Could you check a few things on this drawing? It's one solid part, dimensions in mm from its lowest x, y, z. Coordinates: 2 decimals unless noted, no trailing zeros. Write each loop counter-clockwise with the first axis right and the second up, starting at its lowest first coordinate (ties: lowest second). Pieces come first, ordered by that corner, then holes.
Item 1: I want a section at C-C (z = 1.65). Please give me the cut outline in (x, y), and give its area (3 significant figures).
Item 2: I'm going to push flat-ended pins straight in: P1, Ø1.5, axis at y = 20, z = 0.5, coming from the -X side; P2, Ø2.5, axis at x = 21.4, y = 21.4, coming from the +Z side; P3, Ø6, axis at x = 13, y = 15, coming from the -Z side; P4, Ø1, axis at y = 34.5, z = 3.5, coming from the -X side. Where does each tip first touch, or does it pass through?
Item 3: I want a section at D-D (y = 13). Please give me the cut outline in (x, z), and give its area (3 significant figures).
Item 4: Please list where these lines run through material, in increasing order: line 1 (Y direction, x = 21.4, z = 1.6); line 2 (X direction, y = 29, z = 3.15) (3 decimals); line 3 (X direction, y = 40, z = 3.55).
Item 5: I want a section at A-A (y = 21.4). Please give me the cut outline in (x, z).
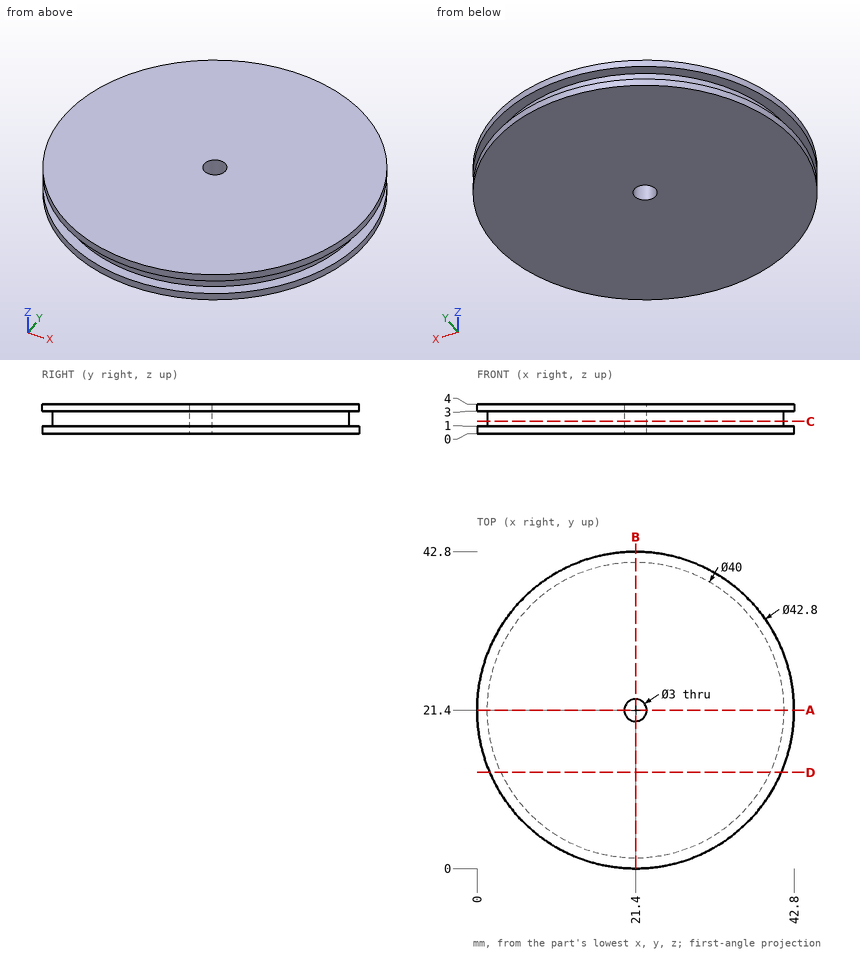
Answer:
1. outline: circle Ø40 at (21.4, 21.4); hole circle Ø3 at (21.4, 21.4)
1. area: 1,250 mm2
2. P1: stops at x = 0.01
2. P2: passes through
2. P3: stops at z = 0
2. P4: stops at x = 4.1
3. outline: (1.72, 0) - (41.08, 0) - (41.08, 1) - (39.55, 1) - (39.55, 3) - (41.08, 3) - (41.08, 4) - (1.72, 4) - (1.72, 3) - (3.25, 3) - (3.25, 1) - (1.72, 1) - close
3. area: 151 mm2
4. line 1: y = 1.4 to 19.9, 22.9 to 41.4
4. line 2: x = 1.395 to 41.405
4. line 3: x = 10.82 to 31.98
5. outline: (0, 0) - (19.9, 0) - (19.9, 4) - (0, 4) - (0, 3) - (1.4, 3) - (1.4, 1) - (0, 1) - close; (22.9, 0) - (42.8, 0) - (42.8, 1) - (41.4, 1) - (41.4, 3) - (42.8, 3) - (42.8, 4) - (22.9, 4) - close
